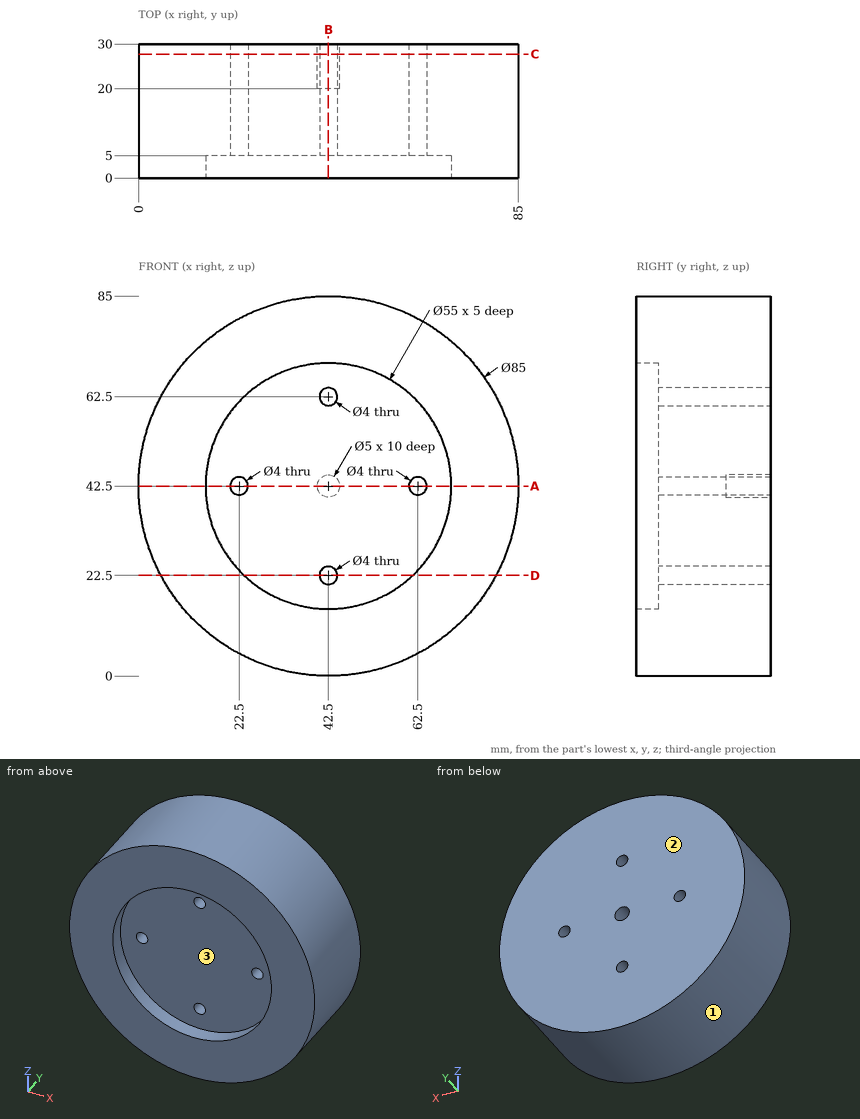
Geometry check sheet. Reference: drawing and pictorial views, mm from the part's lowest x, y, z. Round coordinates to 2 decimals unless told otherwise and drop trailing zeros. Order: outer loops, then holes, each group sorted by start corner. A loop starts at its lowest first (then second) coordinate and runs counter-clockwise, first axis right, second up. Notation, with made-up numbers: (-4.75, -24) - (31.25, -24) arc R20 ccw to (31.25, -19) - close; hole circle Ø8 at (49.25, 30). An arc over 180 degrees is marked (long way). One line per question, with ' | ' between items. Start each with the question number.
(1) Depth check by flat-ended pin: pin 1 Ø1.5 at (y, z) = (23, 49) entering from -X; pin 2 Ø2.5 at (x, z) = (42.5, 62.5) entering from -Y; pin 3 Ø4 at (x, z) = (42.5, 42.5) entering from +Y; pin 4 Ø1 at (x, y) = (48, 14.5) entering from +Z. Enter the tip coordinate at first touch or a pass-through.
(2) Sectioned sample at D-D on z = 22.5. Record the cut outline in (x, y), and give its area (3 significant figures).
(3) Release check for a two-part mould opening along Z. For the marked faces 1, 2 and 3 record: released by +Z, released by -Z, zero draft, split by the parting line, or undercut.
(4) Sectioned sample at A-A on z = 42.5. Record the cut outline in (x, y).
(5) Sectioned sample at C-C on y = 27.75. Record the cut outline in (x, z), and give its area (3 significant figures).
(6) Sectioned sample at B-B on x = 42.5. Record the cut outline in (y, z).
(7) Thickness scan on L1, parallel to X at y = 22.25, z = 42.5; L2, parallel to X at y = 16, z = 42.5; L3, parallel to X at y = 27.75, z = 62.5. Record the ranges inside material, lowest first. Write a range as [from, to].
Conclusion:
1) pin 1: stops at x = 0.39 | pin 2: passes through | pin 3: stops at y = 20 | pin 4: stops at z = 84.7
2) outline: (5, 0) - (23.63, 0) - (23.63, 5) - (40.5, 5) - (40.5, 30) - (5, 30) - close; (44.5, 5) - (61.37, 5) - (61.37, 0) - (80, 0) - (80, 30) - (44.5, 30) - close | area: 1,960 mm2
3) face 1: split by the parting line | face 2: zero draft | face 3: undercut
4) outline: (0, 0) - (15, 0) - (15, 5) - (20.5, 5) - (20.5, 30) - (0, 30) - close; (24.5, 5) - (60.5, 5) - (60.5, 30) - (45, 30) - (45, 20) - (40, 20) - (40, 30) - (24.5, 30) - close; (64.5, 5) - (70, 5) - (70, 0) - (85, 0) - (85, 30) - (64.5, 30) - close
5) outline: circle Ø85 at (42.5, 42.5); hole circle Ø4 at (22.5, 42.5); hole circle Ø5 at (42.5, 42.5); hole circle Ø4 at (42.5, 22.5); hole circle Ø4 at (42.5, 62.5); hole circle Ø4 at (62.5, 42.5) | area: 5,600 mm2
6) outline: (0, 0) - (30, 0) - (30, 20.5) - (5, 20.5) - (5, 15) - (0, 15) - close; (0, 70) - (5, 70) - (5, 64.5) - (30, 64.5) - (30, 85) - (0, 85) - close; (5, 24.5) - (30, 24.5) - (30, 40) - (20, 40) - (20, 45) - (30, 45) - (30, 60.5) - (5, 60.5) - close
7) L1: x = [0, 20.5], [24.5, 40], [45, 60.5], [64.5, 85] | L2: x = [0, 20.5], [24.5, 60.5], [64.5, 85] | L3: x = [5, 40.5], [44.5, 80]
